Autodesk Inventor part; units mm, degrees
ref_plane "YZ Plane" through (0, 0, 0) normal (1, 0, 0) x (0, 1, 0)
ref_plane "XZ Plane" through (0, 0, 0) normal (0, 1, 0) x (-1, 0, 0)
ref_plane "XY Plane" through (0, 0, 0) normal (0, 0, 1) x (1, 0, 0)
sketch "Boceto1" plane through (0, 0, 0) normal (0, 1, 0) x (-1, 0, 0)
  circle A0 centre (0, 0) radius 50
  dimension "Diametro" = 100
extrude "Extrusión1" add sketch "Boceto1" against normal blind 8
fillet "Empalme1" radius 8 1 edges at (50, 0, 0)
sketch "Boceto2" plane through (0, -8, 0) normal (0, -1, 0) x (1, 0, 0)
  circle A0 centre (0, 0) radius 46
  circle A1 centre (0, 0) radius 50
  dimension "d22" = 4
extrude "Extrusión3" add sketch "Boceto2" along normal blind 6 contours A0
sketch "Boceto3" plane through (0, -14, 0) normal (0, -1, 0) x (1, 0, 0)
  point P0 (0, 0)
  point P1 (-37.5, 0)
  point P2 (-18.75, -32.476)
  point P3 (18.75, -32.476)
  point P4 (37.5, 0)
  point P5 (18.75, 32.476)
  point P6 (-18.75, 32.476)
  dimension "d25" = 37.5
  dimension "d35" = 360
hole "Agujero2" at (-37.5, -14, 0) at (-18.75, -14, 32.476) at (-18.75, -14, -32.476) at (18.75, -14, 32.476) at (37.5, -14, 0) at (18.75, -14, -32.476) direction (0, 1, 0) diameter 2.459 depth 8.8
sketch "Boceto4" plane through (0, -14, 0) normal (0, -1, 0) x (1, 0, 0)
  arc A0 (20.5788, -4.4246) -> (20.5788, 4.4246) centre (18.25, 0) ccw
  line L0 (20.5788, 4.4246) -> (6.2877, 11.9463)
  arc A1 (6.2877, 11.9463) -> (-6.2877, 11.9463) centre (0, 0) ccw
  line L1 (-6.2877, 11.9463) -> (-20.5788, 4.4246)
  arc A2 (-20.5788, 4.4246) -> (-20.5788, -4.4246) centre (-18.25, 0) ccw
  line L2 (-20.5788, -4.4246) -> (-6.2877, -11.9463)
  arc A3 (-6.2877, -11.9463) -> (6.2877, -11.9463) centre (0, 0) ccw
  line L3 (6.2877, -11.9463) -> (20.5788, -4.4246)
  line L4 (-17.0094, 4.3256) -> (-5.4726, 10.3977)
  arc A4 (5.4726, 10.3977) -> (-5.4726, 10.3977) centre (0, 0) ccw
  line L5 (5.4726, 10.3977) -> (17.0094, 4.3256)
  arc A5 (17.0094, 4.3256) -> (17.0094, -4.3256) centre (18.25, 0) ccw
  line L6 (17.0094, -4.3256) -> (5.4726, -10.3977)
  arc A6 (-5.4726, -10.3977) -> (5.4726, -10.3977) centre (0, 0) ccw
  line L7 (-5.4726, -10.3977) -> (-17.0094, -4.3256)
  arc A7 (-17.0094, -4.3256) -> (-17.0094, 4.3256) centre (-18.25, 0) ccw
  circle A8 centre (18.25, 0) radius 2.5
  circle A9 centre (-18.25, 0) radius 2.5
  point P0 (0, 0)
  point P1 (20.5788, 4.4246)
  point P2 (-6.2877, 11.9463)
  point P3 (-20.5788, -4.4246)
  point P4 (6.2877, -11.9463)
  dimension "d3" = 8
extrude "Extrusión5" cut sketch "Boceto4" against normal blind 4 contours L3 A3 L2 A2 L1 A1 L0 A0 | L4 A4 L5 A5 L6 A6 L7 A7 | A8 | A9
sketch "Boceto5" plane through (0, -14, 0) normal (0, -1, 0) x (1, 0, 0)
  line L0 (6.2877, 11.9463) -> (20.5788, 4.4246)
  arc A0 (6.2877, 11.9463) -> (-6.2877, 11.9463) centre (0, 0) ccw
  line L1 (-20.5788, 4.4246) -> (-6.2877, 11.9463)
  arc A1 (-20.5788, 4.4246) -> (-20.5788, -4.4246) centre (-18.25, 0) ccw
  line L2 (-6.2877, -11.9463) -> (-20.5788, -4.4246)
  arc A2 (-6.2877, -11.9463) -> (6.2877, -11.9463) centre (0, 0) ccw
  line L3 (20.5788, -4.4246) -> (6.2877, -11.9463)
  arc A3 (20.5788, -4.4246) -> (20.5788, 4.4246) centre (18.25, 0) ccw
  arc A4 (6.4041, 12.1676) -> (-6.4041, 12.1676) centre (0, 0) ccw
  line L4 (6.4041, 12.1676) -> (20.6952, 4.6458)
  arc A5 (20.6952, -4.6458) -> (20.6952, 4.6458) centre (18.25, 0) ccw
  line L5 (20.6952, -4.6458) -> (6.4041, -12.1676)
  arc A6 (-6.4041, -12.1676) -> (6.4041, -12.1676) centre (0, 0) ccw
  line L6 (-6.4041, -12.1676) -> (-20.6952, -4.6458)
  arc A7 (-20.6952, 4.6458) -> (-20.6952, -4.6458) centre (-18.25, 0) ccw
  line L7 (-20.6952, 4.6458) -> (-6.4041, 12.1676)
  point P0 (0, 0)
  dimension "d44" = 0.25
extrude "Extrusión7" cut sketch "Boceto5" against normal up to surface (4 mm away) contours L0 A3 L3 A2 L2 A1 L1 A0 | L4 A5 L5 A6 L6 A7 L7 A4
sketch "Boceto6" plane through (0, 0, 0) normal (0, 1, 0) x (1, 0, 0)
  point P0 (0, 0)
  point P1 (-18.25, 0)
  point P2 (18.25, 0)
hole "Agujero3" at (-18.25, 0, 0) at (18.25, 0, 0) direction (0, -1, 0) diameter 4.134 end through all countersink diameter 10 countersink angle 90
sketch "Boceto7" plane through (0, 0, 0) normal (0, 1, 0) x (1, 0, 0)
  circle A0 centre (0, 0) radius 5
  dimension "d54" = 10
extrude "Extrusión8" cut sketch "Boceto7" against normal through all
sketch "Boceto9" plane through (0, 0, 0) normal (0, 1, 0) x (1, 0, 0)
  circle A0 centre (0, 0) radius 8.0135
  circle A1 centre (0, 0) radius 5
  dimension "d57" = 16.027
  dimension "d58" = 10
extrude "Extrusión9" [suppressed]
extrude "Extrusión10" [suppressed]
properties part number "Tapa" material "Aluminum 7075"
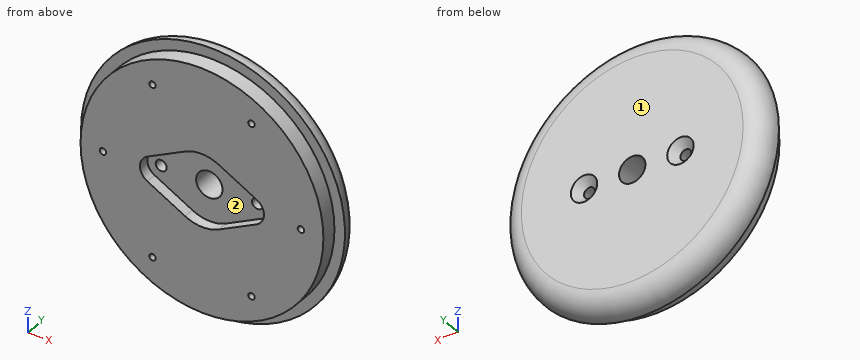
Input: part model. Units: mm. Frame: model coordinates. Face numbers are marked on the shaded views. Give positions to 0.01 mm unless a question says otherwise; leave off trailing zeros. Order: outer loops, then holes, each group sorted by start corner. A loop starts at its lowest first (then second) coordinate and runs counter-clockwise, first axis right, second up. Notation, with made-up numbers: M 28.25,10.25 L 67.25,10.25 A30 cw 67.25,36.25 Z; hole C -3,8 d7. An arc over 180 degrees is marked long. Return JSON: item names as keys, results as strings.
Item 1: Cut plane B-B (z = 0). State how many separate pieces and enclosed holes the cut face has, then the cut area to 3 significant figures.
Solutions:
{"separate pieces": "4", "enclosed holes": "0", "area": "893 mm^2"}
Item 2: First-contact query: P1, Ø2.5, axis at x = 18.5, z = -33, coming from the -Y side; P2, Ø3, axis at y = -3.5, z = 38, coming from the +X side; P3, Ø1.5, axis at x = 18, y = -9.5, coming from the +Z side; P4, Ø9, axis at x = 0, z = 0, coming from the +Y side. Flat tips, straight axial feed; report the tip coordinate or a pass-through.
Solutions:
{"P1": "y = -14", "P2": "x = 32.57", "P3": "z = 42.64", "P4": "through"}
Item 3: Pull-direction query (X, two-part tool) for the marked faces 1 and 2; classes: +X half, -X half, draft (parallel to the pull), parting line (faces both ways), or undercut.
Solutions:
{"face 1": "draft", "face 2": "undercut"}
Item 4: Cut plane A-A (y = -11.5). Return loops of the section in (x, z), then the cut area to 3 significant figures.
Solutions:
{"outline": "C 0,0 d92; hole C -37.5,0 d2.46; hole M -20.7,-4.65 L -6.4,-12.17 A13.75 ccw 6.4,-12.17 L 20.7,-4.65 A5.25 ccw 20.7,4.65 L 6.4,12.17 A13.75 ccw -6.4,12.17 L -20.7,4.65 A5.25 ccw Z; hole C -18.75,-32.48 d2.46; hole C -18.75,32.48 d2.46; hole C 18.75,-32.48 d2.46; hole C 18.75,32.48 d2.46; hole C 37.5,0 d2.46", "area": "5,760 mm^2"}
Item 5: Ray query, probe 1 along Z at (x, y) = (18.75, -8.5); probe 2 along Z at (x, y) = (18.75, -11.25); probe 3 along Y at (x, z) = (-2, -5.5). Return the intervals inside material, ascending.
Solutions:
{"probe 1": "-42.01 to -33.71, -31.25 to -2.01, 2.01 to 31.25, 33.71 to 42.01", "probe 2": "-42.01 to -33.71, -31.25 to -5.67, 5.67 to 31.25, 33.71 to 42.01", "probe 3": "-10 to 0"}
